Input: dimensioned drawing with shaded views. Units: mm. Origin: part minimum x, y, z. Give positions to 0.01 mm unless a question says otherwise; leave off trailing zeros. Write each loop counter-clockwise with the first axis right and the second up, starting at its lowest first coordinate (ties: lowest second). Pieces come first, ordered by that corner, then holes.
Q1. Section C-C (x = 17.5). Return the cut outline in (y, z), plus the area to 3 significant figures.
Q2. Section B-B (y = 14). Return the cut outline in (x, z).
Q3. Pin query (flat end, axial travel): pin 1 Ø1 at (y, z) = (56.5, 1.5) entering from +X; pin 2 Ø1.8 at (x, z) = (23.5, 2.5) entering from -Y; pin 3 Ø1 at (y, z) = (2.5, 1) entering from +X. Return the tip coordinate at first contact, or that it passes through.
Q4. Section A-A (z = 1.4). Return the cut outline in (x, y), plus the area to 4 significant figures.
Q5. Line query: line 1 (Y direction, x = 37, z = 0.8); line 2 (X direction, y = 58, z = 3.05). Output: solid intervals per line, ascending.
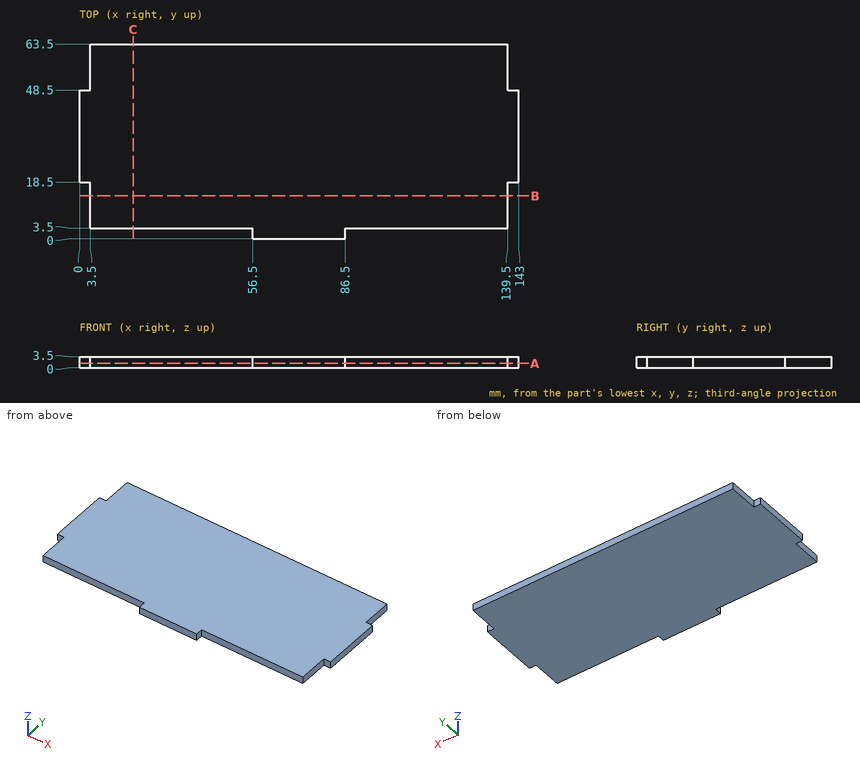
Computed:
1. outline: (3.5, 0) - (63.5, 0) - (63.5, 3.5) - (3.5, 3.5) - close
1. area: 210 mm2
2. outline: (3.5, 0) - (139.5, 0) - (139.5, 3.5) - (3.5, 3.5) - close
3. pin 1: stops at x = 139.5
3. pin 2: stops at y = 3.5
3. pin 3: stops at x = 86.5
4. outline: (0, 18.5) - (3.5, 18.5) - (3.5, 3.5) - (56.5, 3.5) - (56.5, 0) - (86.5, 0) - (86.5, 3.5) - (139.5, 3.5) - (139.5, 18.5) - (143, 18.5) - (143, 48.5) - (139.5, 48.5) - (139.5, 63.5) - (3.5, 63.5) - (3.5, 48.5) - (0, 48.5) - close
4. area: 8,475 mm2
5. line 1: y = 3.5 to 63.5
5. line 2: x = 3.5 to 139.5
